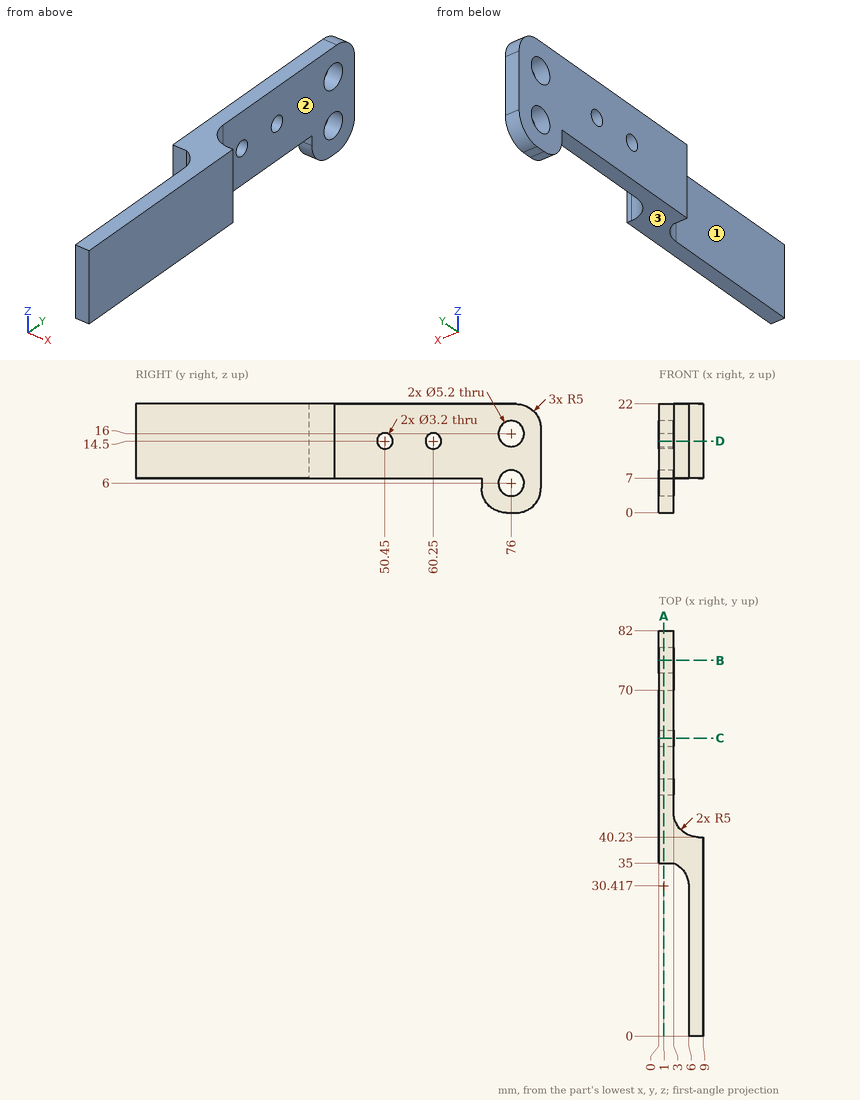
Part print with two shaded views. Sizes in mm from the minimum x, y, z corner. A direction names the side the tool comes from. Coordinates: 2 decimals unless noted, no trailing zeros. Order: outer loops, then holes, each group sorted by start corner. A loop starts at its lowest first (then second) coordinate and runs counter-clockwise, first axis right, second up. Notation, with made-up numbers: (6.25, 72.25) - (21.25, 72.25) arc R22 ccw to (21.25, 108.25) - close; hole circle Ø8 at (-37, 0). An arc over 180 degrees is marked (long way). Write item = value, one per line. Start each with the question number.
1) Wall check: line 1 along Z through (x, y) = (0.6, 60.25); line 2 along X through (y, z) = (12, 8.5); line 3 along Z through (x, y) = (7.25, 24). Give the ranges that are in metal, low to high. Write a range as from..to.
2) Saw through at C-C on y = 60.25. Write the cut outline in (x, z).
3) Saw through at B-B on y = 76. Write the cut outline in (x, z).
4) Saw through at A-A on x = 1. Write the cut outline in (y, z).
5) Flat gauge pins, fed straight in: pin 1 Ø0.8 at (x, z) = (8.5, 17.5) entering from +Y; pin 2 Ø10 at (y, z) = (68.5, 15) entering from +X; pin 3 Ø4.5 at (y, z) = (13, 17.5) entering from -X. Where does each tip first touch, or does it go through?
6) 3-axis set-ups, long thin cutter, end or side, ignore diameter. For the marked faces 1, 2 and 3: which of +Z, -Z, +X, -X, +Y, -Y reach the whole face in a straight line?
7) Saw through at D-D on z = 14.5. Write the cut outline in (x, y).
From the geometry:
q1.line_1 = 7..12.9, 16.1..22
q1.line_2 = 6..9
q1.line_3 = 7..22
q2.outline = (0, 7) - (3, 7) - (3, 12.9) - (0, 12.9) - close; (0, 16.1) - (3, 16.1) - (3, 22) - (0, 22) - close
q3.outline = (0, 0) - (3, 0) - (3, 3.4) - (0, 3.4) - close; (0, 8.6) - (3, 8.6) - (3, 13.4) - (0, 13.4) - close; (0, 18.6) - (3, 18.6) - (3, 22) - (0, 22) - close
q4.outline = (35, 7) - (70, 7) - (70, 5) arc R5 ccw to (75, 0) - (77, 0) arc R5 ccw to (82, 5) - (82, 17) arc R5 ccw to (77, 22) - (35, 22) - close; hole circle Ø3.2 at (50.45, 14.5); hole circle Ø3.2 at (60.25, 14.5); hole circle Ø5.2 at (76, 6); hole circle Ø5.2 at (76, 16)
q5.pin_1 = 40.23
q5.pin_2 = 3
q5.pin_3 = 6
q6.face_1 = +Z, -Z, -X, -Y
q6.face_2 = +Z, -Z, +X, +Y
q6.face_3 = -Z, +X, -X, -Y
q7.outline = (0, 35) - (3, 35) arc R5 cw to (6, 30.42) - (6, 0) - (9, 0) - (9, 40.23) - (8, 40.23) arc R5 cw to (3, 45.23) - (3, 48.85) - (0, 48.85) - close; (0, 52.05) - (3, 52.05) - (3, 58.65) - (0, 58.65) - close; (0, 61.85) - (3, 61.85) - (3, 73.88) - (0, 73.88) - close; (0, 78.12) - (3, 78.12) - (3, 82) - (0, 82) - close
